Part model, mm, in its own coordinate system. A direction names the side the tool comes from. Coordinates: 2 decimals unless noted, no trailing zeros. Order: outer loops, then holes, each group sorted by start corner. A loop starts at its lowest first (then second) coordinate and runs counter-clockwise, first axis right, second up.
from build123d import *

# Parameters (mm, degrees)
SKETCH1_W           = 40
SKETCH1_H           = 40
BOSS_EXTRUDE1_DEPTH = 50
SKETCH2_R           = 10.65
CUT_EXTRUDE1_DEPTH  = 58.445626465
SKETCH3_W           = 20.063984789
SKETCH3_H           = 19.357087105
BOSS_EXTRUDE2_DEPTH = 20
SKETCH4_R           = 3.619370809
BOSS_EXTRUDE3_DEPTH = 10


with BuildPart() as part:
    # Sketch1 → Boss-Extrude1 (new body)
    with BuildSketch(Plane.XY):
        Rectangle(SKETCH1_W, SKETCH1_H)
    extrude(amount=BOSS_EXTRUDE1_DEPTH)

    # Sketch2 → Cut-Extrude1 (cut, through all)
    with BuildSketch(Plane.XY.offset(50)):
        Circle(SKETCH2_R)
    extrude(amount=-CUT_EXTRUDE1_DEPTH, mode=Mode.SUBTRACT)

    # Sketch3 → Boss-Extrude2 (add)
    with BuildSketch(Plane(origin=(0, 20, 0), x_dir=(1, 0, 0), z_dir=(0, 1, 0))):
        with Locations((-1.432326622, -18.882716681)):
            Rectangle(SKETCH3_W, SKETCH3_H)
    extrude(amount=BOSS_EXTRUDE2_DEPTH)

    # Sketch4 → Boss-Extrude3 (add)
    with BuildSketch(Plane(origin=(0, 0, 9.204173129), x_dir=(-1, 0, 0), z_dir=(0, 0, -1))):
        with Locations(Location((1.944917796, 31.214146172, 0), (0, 0, 180))):
            Circle(SKETCH4_R)
    extrude(amount=BOSS_EXTRUDE3_DEPTH)


solid = part.part
Q1. Cut at A-A on y = 0. Write the cut outline in (x, z), and give its area (3 significant figures).
Results list:
outline: (-20, 0) - (-10.65, 0) - (-10.65, 50) - (-20, 50) - close; (10.65, 0) - (20, 0) - (20, 50) - (10.65, 50) - close
area: 935 mm2
Q2. Cut at B-B on z = 16. Write the cut outline in (x, y).
Results list:
outline: (-20, -20) - (20, -20) - (20, 20) - (8.6, 20) - (8.6, 40) - (-11.46, 40) - (-11.46, 20) - (-20, 20) - close; hole circle Ø21.3 at (0, 0)
Q3. Cut at C-C on x = 3. Write the cut outline in (y, z), and give its area (3 significant figures).
Results list:
outline: (-20, 0) - (-10.22, 0) - (-10.22, 50) - (-20, 50) - close; (10.22, 0) - (20, 0) - (20, 9.2) - (40, 9.2) - (40, 28.56) - (20, 28.56) - (20, 50) - (10.22, 50) - close
area: 1,370 mm2
Q4. Mould opens along X. For faces 1 (the face through (-2.416, 27.626, 4.274)), 2 (the face through (0, -20, 25)), 3 (the face through (-11.464, 30, 19)), 4 (the face through (10.158, 3.199, 25.35)) say: pulls with the +X half, pulls with the -X half, needs draft (parallel to the pull), parting line crosses it, or undercut.
Results list:
face 1: parting line crosses it
face 2: needs draft
face 3: pulls with the -X half
face 4: undercut
Q5. Wall check: line 1 along Y through (x, z) = (0, 27); line 2 along Y through (x, z) = (1, 2); line 3 along Y through (x, z) = (0, 35.5). Give the ranges that are in metal, low to high.
Results list:
line 1: y = -20 to -10.65, 10.65 to 40
line 2: y = -20 to -10.6, 10.6 to 20, 29.11 to 33.32
line 3: y = -20 to -10.65, 10.65 to 20
Q6. Pin check, flat tips, straight feed: pin 1 Ø1.5 at (x, z) = (-6, 35) entering from +Y; pin 2 Ø6 at (x, y) = (-5, 10.5) entering from -Z; pin 3 Ø9.5 at (y, z) = (33, 21) entering from +X; pin 4 Ø6 at (x, y) = (-2, 25.5) entering from -Z. Stop position of each tip, or through.
Results list:
pin 1: stops at y = 20
pin 2: stops at z = 0
pin 3: stops at x = 8.6
pin 4: stops at z = -0.8
Q7. Which spindle directions (+Z, -Z, +X, -X, +Y, -Y) get a long thin tool onto all of the face, cutting with end or side? Do faces 5 (the face through (1, 28, 9.204)), 6 (the face through (-2, 30, 28.561)), 7 (the face through (9, 9, 0)), 8 (the face through (8.6, 30, 19)). Say none if no direction does.
Results list:
face 5: -Z
face 6: +Z, +X, -X, +Y
face 7: -Z, +X, -X, -Y
face 8: +Z, -Z, +X, +Y
Q8. Cut at D-D on z = 7. Write the cut outline in (x, y), and give its area (3 significant figures).
Results list:
outline: (-20, -20) - (20, -20) - (20, 20) - (-20, 20) - close; circle Ø7.24 at (-1.94, 31.21); hole circle Ø21.3 at (0, 0)
area: 1,280 mm2
